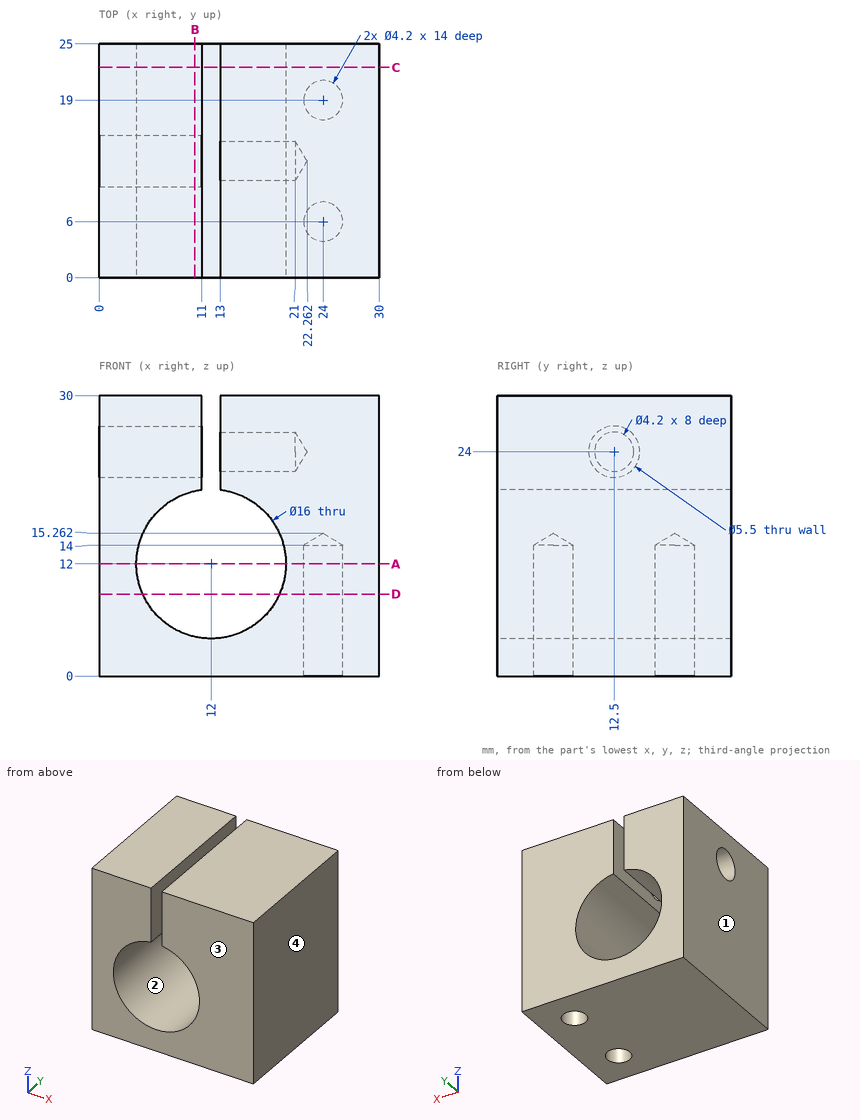
Answer from the drawing. Dimensions are ordinates in mm from the lowest x, y and z of the part. Round coordinates to 2 decimals unless told otherwise and drop trailing zeros. Write each loop counter-clockwise with the first axis right and the second up, starting at its lowest first coordinate (ties: lowest second). Pieces come first, ordered by that corner, then holes. Notation, with made-up numbers: (59, 5.5) - (103, 5.5) arc R17 cw to (103, 31.5) - close; hole circle Ø9 at (-9.5, 36.25). An arc over 180 degrees is marked (long way). One line per item, written item: value.
Q1. For a pull along X with two mould halves and no side action, classify the marked faces 1, 2, 3 and 4 as pulls with the +X half, pulls with the -X half, needs draft (parallel to the pull), parting line crosses it, or undercut.
The answers:
face 1: pulls with the -X half
face 2: undercut
face 3: needs draft
face 4: pulls with the +X half
Q2. Find section B-B (x = 10.25). Determine the outline of the cut face in (y, z).
The answers:
outline: (0, 0) - (25, 0) - (25, 4.19) - (0, 4.19) - close; (0, 19.81) - (25, 19.81) - (25, 30) - (0, 30) - close; hole circle Ø5.5 at (12.5, 24)
Q3. Each of these flat-tipped pins is pushed along its axis until it touches: P1, Ø3.5, axis at x = 24, y = 19, coming from the -Z side; P2, Ø4, axis at y = 12.5, z = 24, coming from the -X side. Where does it stop, or does it pass through?
The answers:
P1: stops at z = 14.21
P2: stops at x = 21.06
Q4. Find section A-A (z = 12). Determine the outline of the cut face in (x, y), and give its area (3 significant figures).
The answers:
outline: (0, 0) - (4, 0) - (4, 25) - (0, 25) - close; (20, 0) - (30, 0) - (30, 25) - (20, 25) - close; hole circle Ø4.2 at (24, 6); hole circle Ø4.2 at (24, 19)
area: 322 mm2
Q5. Straight lines are drawn through the part: line 1 (Y direction, x = 24, z = 6.5); line 2 (Y direction, x = 18.5, z = 24); line 3 (X direction, y = 14, z = 12). For each, find the intervals that lie inside material, in ascending order. Write a range as from..to.
The answers:
line 1: y = 0..3.9, 8.1..16.9, 21.1..25
line 2: y = 0..10.4, 14.6..25
line 3: x = 0..4, 20..30
Q6. Find section C-C (y = 22.5). Determine the outline of the cut face in (x, z), and give its area (3 significant figures).
The answers:
outline: (0, 0) - (30, 0) - (30, 30) - (13, 30) - (13, 19.94) arc R8 cw (long way) to (11, 19.94) - (11, 30) - (0, 30) - close
area: 679 mm2
Q7. Find section D-D (z = 8.75). Determine the outline of the cut face in (x, y), and give its area (3 significant figures).
The answers:
outline: (0, 0) - (4.69, 0) - (4.69, 25) - (0, 25) - close; (19.31, 0) - (30, 0) - (30, 25) - (19.31, 25) - close; hole circle Ø4.2 at (24, 6); hole circle Ø4.2 at (24, 19)
area: 357 mm2
